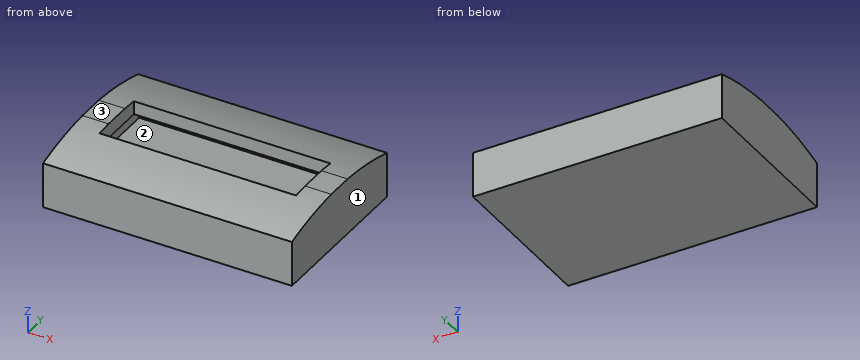
```python
from build123d import *

# Parameters (mm, degrees)
CROQUIS1_W              = 380
CROQUIS1_H              = 250
SALIENTE_EXTRUIR1_DEPTH = 64
CROQUIS2_W              = 372
CROQUIS2_H              = 242
CORTAR_EXTRUIR1_DEPTH   = 60
CROQUIS3_W              = 380
CROQUIS3_H              = 250
SALIENTE_EXTRUIR2_DEPTH = 22
CROQUIS5_W              = 300
CROQUIS5_H              = 90
CORTAR_EXTRUIR3_DEPTH   = 41
CORTAR_EXTRUIR2_REACH   = 411.171


with BuildPart() as part:
    # Croquis1 → Saliente-Extruir1 (new body)
    with BuildSketch(Plane.XY):
        Rectangle(CROQUIS1_W, CROQUIS1_H)
    extrude(amount=SALIENTE_EXTRUIR1_DEPTH)

    # Croquis2 → Cortar-Extruir1 (cut)
    with BuildSketch(Plane.XY.offset(64)):
        Rectangle(CROQUIS2_W, CROQUIS2_H)
    extrude(amount=-CORTAR_EXTRUIR1_DEPTH, mode=Mode.SUBTRACT)

    # Croquis3 → Saliente-Extruir2 (add)
    with BuildSketch(Plane.XY.offset(64)):
        Rectangle(CROQUIS3_W, CROQUIS3_H)
    extrude(amount=SALIENTE_EXTRUIR2_DEPTH)

    # Croquis5 → Cortar-Extruir3 (cut)
    with BuildSketch(Plane.XY.offset(86)):
        Rectangle(CROQUIS5_W, CROQUIS5_H)
    extrude(amount=-CORTAR_EXTRUIR3_DEPTH, mode=Mode.SUBTRACT)

    # Cortar-Extruir2: up to this face of the body (flat: up to its plane)
    cortar_extruir2_end = Plane(part.part.faces().sort_by_distance((190, 0, 43))[0])
    # Croquis4 → Cortar-Extruir2 (cut, up to the picked face)
    with BuildSketch(Plane.ZY.offset(190), mode=Mode.PRIVATE) as cortar_extruir2_sk1:
        with BuildLine():
            Line((69, 125), (69, 152.478721162))
            Line((69, 152.478721162), (170.671845975, 152.478721162))
            Line((170.671845975, 152.478721162), (170.671845975, -144.88621918))
            Line((170.671845975, -144.88621918), (69, -144.88621918))
            Line((69, -144.88621918), (69, -125))
            ThreePointArc((69, -125), (86.50817069, 0), (69, 125))
        make_face()
    cortar_extruir2_tool1 = split(extrude(cortar_extruir2_sk1.sketch, amount=-CORTAR_EXTRUIR2_REACH, mode=Mode.PRIVATE), bisect_by=cortar_extruir2_end, keep=Keep.BOTH, mode=Mode.PRIVATE)
    add(cortar_extruir2_tool1.solids().sort_by(Axis((-190, 4.203548, 124.537441), (1, 0, 0)))[0], mode=Mode.SUBTRACT)


solid = part.part
```
Could you check a few things on this model? Use its own coordinates, in mm. Face numbers are marked on the shaded views. Coordinates: 2 decimals unless noted, no trailing zeros. Loops run counter-clockwise (first coordinate to the right, second up) from the corner with the lowest first, then second, coordinate; pieces in that order, holes last.
1) Imagine slicing it at A-A (x = -163). List the corners of the cut face in (y, z) for me.
Reported:
outline: (-125, 0) - (125, 0) - (125, 69) arc R454.97 ccw to (21.5, 86) - (-21.5, 86) arc R454.97 ccw to (-125, 69) - close; hole (-121, 4) - (121, 4) - (121, 64) - (-121, 64) - close
2) Imagine slicing it at D-D (x = 30). List the corners of the cut face in (y, z) for me, and give its area (3 significant figures).
Reported:
outline: (-125, 0) - (125, 0) - (125, 69) arc R454.97 ccw to (45, 84.28) - (45, 64) - (121, 64) - (121, 4) - (-121, 4) - (-121, 64) - (-45, 64) - (-45, 84.28) arc R454.97 ccw to (-125, 69) - close
area: 3,700 mm2
3) Imagine slicing it at C-C (z = 21). List the corners of the cut face in (x, y) for me, and give its area (3 significant figures).
Reported:
outline: (-190, -125) - (190, -125) - (190, 125) - (-190, 125) - close; hole (-186, -121) - (186, -121) - (186, 121) - (-186, 121) - close
area: 4,980 mm2
4) Please list where these lines run through material, in increasing order: line 1 along Y through (x, z) = (-127, 20.5); line 2 along X through (y, z) = (-61, 7); line 3 along Z through (x, y) = (-161.5, -15.5).
Reported:
line 1: y = -125 to -121, 121 to 125
line 2: x = -190 to -186, 186 to 190
line 3: z = 0 to 4, 64 to 86
5) Will these pins go through, and if not, where does the flat tip stop? pin 1 Ø3 at (x, y) = (-148, -97) entering from +Z; pin 2 Ø10 at (x, z) = (-5, 69.5) entering from -Y; pin 3 Ø5 at (x, y) = (87, 17.5) entering from +Z; pin 4 Ø2 at (x, y) = (-12.5, -79.5) entering from +Z.
Reported:
pin 1: stops at z = 76.37
pin 2: stops at y = -125
pin 3: stops at z = 4
pin 4: stops at z = 79.68
6) Thinking about a two-plate mould opening in Z: for the marked faces 1, 2 and 3, which applies, released by +Z, released by -Z, zero draft, split by the parting line, or undercut?
Reported:
face 1: zero draft
face 2: undercut
face 3: released by +Z
7) Imagine slicing it at B-B (y = 65). List the corners of the cut face in (x, z) for me.
Reported:
outline: (-190, 0) - (190, 0) - (190, 81.84) - (-190, 81.84) - close; hole (-186, 4) - (186, 4) - (186, 64) - (-186, 64) - close
